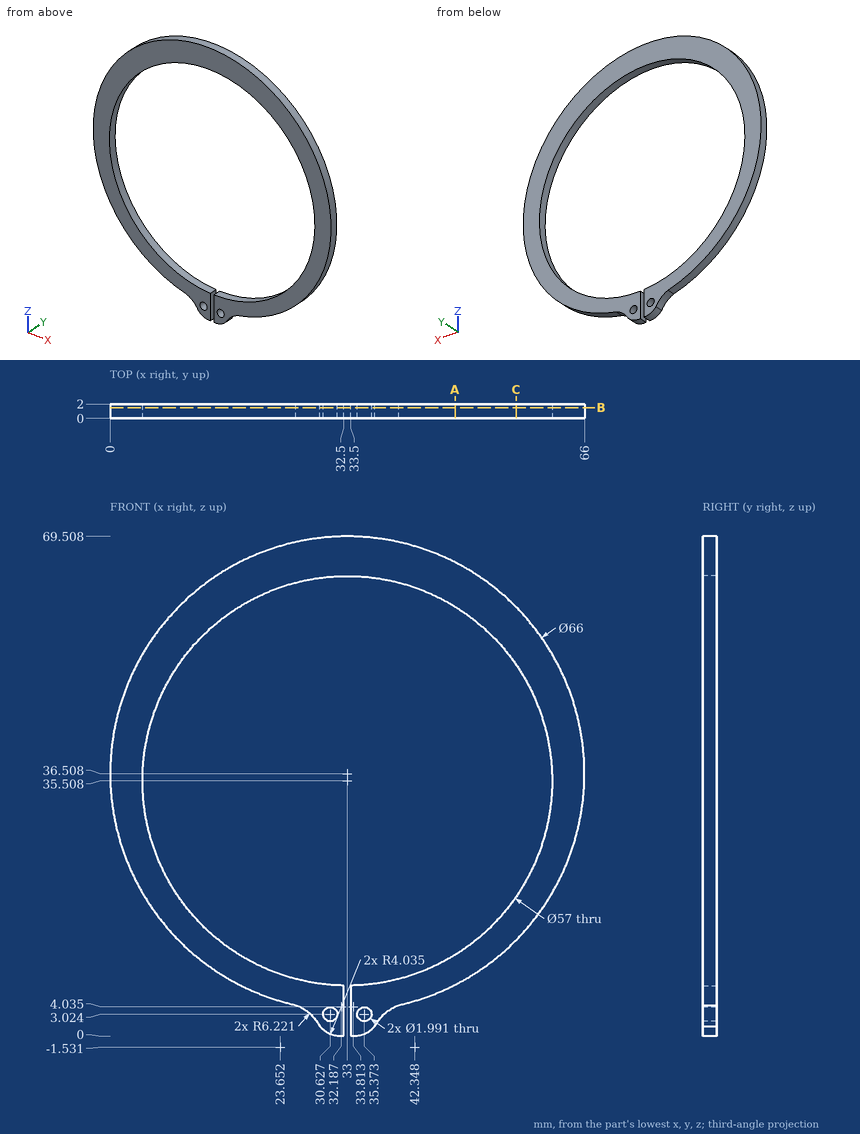
Geometry check sheet. Reference: drawing and pictorial views, mm from the part's lowest x, y, z. Give positions to 0.01 mm unless a question says otherwise; leave off trailing zeros. Loops run counter-clockwise (first coordinate to the right, second up) from the corner with the lowest first, then second, coordinate; pieces in that order, holes last.
1. Section check B-B, the plane y = 1.5. Enter the section's corners in (x, z) (1 decimal).
2. Thickness scan on line 1 (X direction, y = 0.8, z = 3) (1 decimal); line 2 (Z direction, x = 22, y = 1.5) (1 decimal); line 3 (X direction, y = 1.05, z = 10) (1 decimal). Record the ranges inside material, lowest first.
3. Section check C-C, the plane x = 56.5. Enter the section's corners in (y, z) (1 decimal).
4. Section check A-A, the plane x = 48. Enter the section's corners in (y, z) (1 decimal).
5. Go/stop test with flat-tipped pins: pin 1 Ø1 at (y, z) = (0.5, 37.5) entering from -X; pin 2 Ø1.6 at (x, z) = (30.63, 3.02) entering from -Y (3 decimals); pin 3 Ø1 at (y, z) = (0.5, 16) entering from -X. Record where each tip stops, or that it passes through.
Geometry says:
1. outline: (25.8, 4.3) arc R6.2 cw to (29.2, 1.4) arc R4 ccw to (32.5, 0) - (32.5, 7) arc R28.5 cw (long way) to (33.5, 7) - (33.5, 0) arc R4 ccw to (36.8, 1.4) arc R6.2 cw to (40.2, 4.3) arc R33 ccw (long way) to start; hole circle Ø2 at (30.6, 3); hole circle Ø2 at (35.4, 3)
2. line 1: x = 27.9 to 29.6, 31.6 to 32.5, 33.5 to 34.4, 36.4 to 38.1
2. line 2: z = 5.4 to 9.2, 61.8 to 67.6
2. line 3: x = 13.3 to 20.3, 45.7 to 52.7
3. outline: (0, 13.3) - (2, 13.3) - (2, 19.4) - (0, 19.4) - close; (0, 51.6) - (2, 51.6) - (2, 59.7) - (0, 59.7) - close
4. outline: (0, 7.1) - (2, 7.1) - (2, 11.3) - (0, 11.3) - close; (0, 59.7) - (2, 59.7) - (2, 65.9) - (0, 65.9) - close
5. pin 1: stops at x = 0
5. pin 2: passes through
5. pin 3: stops at x = 6.76
